from build123d import *

# Parameters (mm, degrees)
TUBE_R          = 7.5
TUBE_R_2        = 4
TUBE_DEPTH      = 6.5
FILLET004_1_R   = 1.6
FILLET004_2_R   = 0.4
SKETCH014_R     = 12.203108
POCKET005_DEPTH = 6.501


with BuildPart() as part:
    # Tube → Tube (new body)
    with BuildSketch(Plane.XY):
        Circle(TUBE_R)
        Circle(TUBE_R_2, mode=Mode.SUBTRACT)
    extrude(amount=TUBE_DEPTH)

    # Fillet004 1
    fillet004_1_edges = [part.edges().sort_by_distance(p)[0] for p in [
        (-7.5, 0, 6.5),
        (-7.5, 0, 0),
    ]]
    fillet(fillet004_1_edges, radius=FILLET004_1_R)

    # Fillet004 2
    fillet004_2_edges = [part.edges().sort_by_distance(p)[0] for p in [
        (-4, 0, 6.5),
        (-4, 0, 0),
    ]]
    fillet(fillet004_2_edges, radius=FILLET004_2_R)

    # Sketch014 → Pocket005 (cut, through all)
    with BuildSketch(Plane.XY):
        Circle(SKETCH014_R)
        Polygon((6.5, -3.752777), (6.5, 3.752777), (0, 7.505553), (-6.5, 3.752777), (-6.5, -3.752777), (0, -7.505553), align=None, mode=Mode.SUBTRACT)
    extrude(amount=POCKET005_DEPTH, mode=Mode.SUBTRACT)


solid = part.part
Read the model definition and answer for the solid it produces. Units are mm, in the model's axes. Round coordinates to 2 decimals unless told otherwise and drop trailing zeros. Write each loop counter-clockwise with the first axis right and the second up, starting at its lowest first coordinate (ties: lowest second). Pieces come first, ordered by that corner, then holes. Notation, with made-up numbers: (69.25, 39.5) - (105.25, 39.5) arc R25 cw to (105.25, 54.5) - close; hole circle Ø4 at (-16, 13.25). An arc over 180 degrees is marked (long way). Use a Markdown table: item, result.
(1) The part is cut by section C-C (z = 1.25). Write down the section's boundary in (x, y).
Reported:
| item | result |
|---|---|
| outline | (-6.5, -3.66) arc R7.46 ccw to (-6.42, -3.8) - (-0.08, -7.46) arc R7.46 ccw to (0.08, -7.46) - (6.42, -3.8) arc R7.46 ccw to (6.5, -3.66) - (6.5, 3.66) arc R7.46 ccw to (6.42, 3.8) - (0.08, 7.46) arc R7.46 ccw to (-0.08, 7.46) - (-6.42, 3.8) arc R7.46 ccw to (-6.5, 3.66) - close; hole circle Ø8 at (0, 0) |
(2) Each of these flat-tipped pins is pushed along its axis until it touches: pin 1 Ø1.5 at (x, z) = (-1, 2.5) entering from -Y; pin 2 Ø3 at (x, z) = (2.5, 4) entering from -Y. Where does it stop, or does it pass through?
Reported:
| item | result |
|---|---|
| pin 1 | y = -7.36 |
| pin 2 | y = -6.93 |
(3) The mould has two halves that part along X. Classify faces 1 (the flat face through (-6.5, 0, 3)), 2 (the cylindrical face through (-0.867, -3.905, 3.21)), 3 (the flat face through (-4, -2.2, 0)), 4 (the flat face through (3.2, -5.66, 3.21)): released by +X, released by -X, zero draft, split by the parting line, or undercut.
Reported:
| item | result |
|---|---|
| face 1 | released by -X |
| face 2 | undercut |
| face 3 | zero draft |
| face 4 | released by +X |
(4) The part is cut by section A-A (y = 0). Write down the section's boundary in (x, z), then the cut area to 3 significant figures.
Reported:
| item | result |
|---|---|
| outline | (-6.5, 0.12) arc R1.6 ccw to (-5.9, 0) - (-4.4, 0) arc R0.4 ccw to (-4, 0.4) - (-4, 6.1) arc R0.4 ccw to (-4.4, 6.5) - (-5.9, 6.5) arc R1.6 ccw to (-6.5, 6.38) - close; (4, 0.4) arc R0.4 ccw to (4.4, 0) - (5.9, 0) arc R1.6 ccw to (6.5, 0.12) - (6.5, 6.38) arc R1.6 ccw to (5.9, 6.5) - (4.4, 6.5) arc R0.4 ccw to (4, 6.1) - close |
| area | 32.3 mm2 |
(5) Straight lines are drawn through the part: line 1 along Z through (x, y) = (3.5, -2.5); line 2 along Y through (x, z) = (-3, 4.5); line 3 along X through (y, z) = (1.25, 0.5). For each, find the intervals that lie inside material, in ascending order. Write a range as [from, to].
Reported:
| item | result |
|---|---|
| line 1 | [0.01, 6.49] |
| line 2 | [-5.77, -2.65], [2.65, 5.77] |
| line 3 | [-6.5, -3.8], [3.8, 6.5] |
